from build123d import *

# Parameters (mm, degrees)
SKETCH1_R           = 10
BOSS_EXTRUDE1_DEPTH = 175
CHAMFER2_SIZE       = 0.5
SKETCH2_R           = 3
CUT_EXTRUDE1_DEPTH  = 20
CHAMFER3_SIZE       = 0.5
SKETCH3_R           = 3
CUT_EXTRUDE2_DEPTH  = 20
SKETCH4_R           = 10
SKETCH4_R_2         = 5
CUT_EXTRUDE3_DEPTH  = 273
CHAMFER5_SIZE       = 0.5


with BuildPart() as part:
    # Sketch1 → Boss-Extrude1 (new body)
    with BuildSketch(Plane(origin=(0, 0, 0), x_dir=(1, 0, 0), z_dir=(0, 1, 0))):
        Circle(SKETCH1_R)
    extrude(amount=BOSS_EXTRUDE1_DEPTH)

    # Chamfer2
    chamfer2_edges = [part.edges().sort_by_distance(p)[0] for p in [
        (-10, 0, 0),
        (-10, 175, 0),
    ]]
    chamfer(chamfer2_edges, length=CHAMFER2_SIZE)

    # Sketch2 → Cut-Extrude1 (cut)
    with BuildSketch(Plane(origin=(0, 175, 0), x_dir=(1, 0, 0), z_dir=(0, 1, 0))):
        Circle(SKETCH2_R)
    extrude(amount=-CUT_EXTRUDE1_DEPTH, mode=Mode.SUBTRACT)

    # Chamfer3
    chamfer3_edges = [part.edges().sort_by_distance(p)[0] for p in [
        (-3, 175, 0),
    ]]
    chamfer(chamfer3_edges, length=CHAMFER3_SIZE)

    # Sketch3 → Cut-Extrude2 (cut)
    with BuildSketch(Plane.XZ):
        Circle(SKETCH3_R)
    extrude(amount=-CUT_EXTRUDE2_DEPTH, mode=Mode.SUBTRACT)

    # Sketch4 → Cut-Extrude3 (cut)
    with BuildSketch(Plane.XZ):
        Circle(SKETCH4_R)
        Circle(SKETCH4_R_2, mode=Mode.SUBTRACT)
    extrude(amount=-CUT_EXTRUDE3_DEPTH, mode=Mode.SUBTRACT)

    # Chamfer5
    chamfer5_edges = [part.edges().sort_by_distance(p)[0] for p in [
        (-3, 0, 0),
        (-5, 175, 0),
        (-5, 0, 0),
    ]]
    chamfer(chamfer5_edges, length=CHAMFER5_SIZE)


solid = part.part
Source: CAD feature listing. Evaluate the final solid. Frame: model axes, mm. A direction names the side the tool comes from. Coordinates: 2 decimals unless noted, no trailing zeros. Order: outer loops, then holes, each group sorted by start corner. A loop starts at its lowest first (then second) coordinate and runs counter-clockwise, first axis right, second up.
Item 1: Cut plane A-A (z = 0). Return loops of the section in (x, y).
Output values:
outline: (-5, 0.5) - (-4.5, 0) - (-3.5, 0) - (-3, 0.5) - (-3, 20) - (3, 20) - (3, 0.5) - (3.5, 0) - (4.5, 0) - (5, 0.5) - (5, 174.5) - (4.5, 175) - (3.5, 175) - (3, 174.5) - (3, 155) - (-3, 155) - (-3, 174.5) - (-3.5, 175) - (-4.5, 175) - (-5, 174.5) - close
Item 2: Pull-direction query (X, two-part tool) for faces 4 (the face through (0, 0, 4)), 5 (the face through (-3, 165, 0)), 6 (the face through (-1.08, 86.28, -4.88)); classes: pulls with the +X half, pulls with the -X half, needs draft (parallel to the pull), parting line crosses it, or undercut.
Output values:
face 4: needs draft
face 5: undercut
face 6: parting line crosses it
Item 3: Material intervals for line 1 (Z direction, x = 0, y = 9.5); line 2 (Y direction, x = -2, z = -2); line 3 (X direction, y = 11.5, z = 2), sorted ascending.
Output values:
line 1: z = -5 to -3, 3 to 5
line 2: y = 20 to 155
line 3: x = -4.58 to -2.24, 2.24 to 4.58
Item 4: Cut plane C-C (y = 112). Return loops of the section in (x, z), plus the area to 3 significant figures.
Output values:
outline: circle Ø10 at (0, 0)
area: 78.5 mm2
Item 5: First-contact query: P1, Ø5.5, axis at x = 0, z = 0, coming from the -Y side; P2, Ø3, axis at x = -2, y = 81.5, coming from the -Z side; P3, Ø1, axis at x = 1.5, y = 28, coming from the -Z side. Flat tips, straight axial feed; report the tip coordinate or a pass-through.
Output values:
P1: stops at y = 20
P2: stops at z = -4.97
P3: stops at z = -4.9
Item 6: Cut plane B-B (x = 0). Return loops of the section in (y, z).
Output values:
outline: (0, -4.5) - (0.5, -5) - (174.5, -5) - (175, -4.5) - (175, -3.5) - (174.5, -3) - (155, -3) - (155, 3) - (174.5, 3) - (175, 3.5) - (175, 4.5) - (174.5, 5) - (0.5, 5) - (0, 4.5) - (0, 3.5) - (0.5, 3) - (20, 3) - (20, -3) - (0.5, -3) - (0, -3.5) - close
Item 7: Set-up query: faces 1 (the face through (-3, 10, 0)), 2 (the face through (0, 155, 0)), 3 (the face through (0, 175, 4)). Return all of +Z, -Z, +X, -X, +Y, -Y with unobstructed straight access to the full face (end or side cutting, diameter ignored); none if empty.
Output values:
face 1: -Y
face 2: +Y
face 3: +Z, -Z, +X, -X, +Y
